Read the model definition and answer for the solid it produces. Units are mm, in the model's axes. Round coordinates to 2 decimals unless told otherwise and drop trailing zeros. Write each loop counter-clockwise with the first axis right and the second up, starting at its lowest first coordinate (ties: lowest second). Pieces come first, ordered by that corner, then holes.
from build123d import *

# Parameters (mm, degrees)
SKETCH1_W           = 76.2
SKETCH1_H           = 288.925
BOSS_EXTRUDE1_DEPTH = 3.175
CUT_EXTRUDE1_REACH  = 300.821
SKETCH2_W           = 65.532
SKETCH2_H           = 96.012


with BuildPart() as part:
    # Sketch1 → Boss-Extrude1 (new body)
    with BuildSketch(Plane(origin=(0, 0, 0), x_dir=(0, 0, -1), z_dir=(1, 0, 0))):
        with Locations((38.1, 144.4625)):
            Rectangle(SKETCH1_W, SKETCH1_H)
    extrude(amount=BOSS_EXTRUDE1_DEPTH)

    # Sketch2 → Cut-Extrude1 (cut, up to next)
    with BuildSketch(Plane.ZY, mode=Mode.PRIVATE) as cut_extrude1_sk1:
        with Locations((-38.1, 234.569)):
            Rectangle(SKETCH2_W, SKETCH2_H)
    cut_extrude1_tool1 = extrude(cut_extrude1_sk1.sketch, amount=-CUT_EXTRUDE1_REACH, mode=Mode.PRIVATE) & part.part
    add(cut_extrude1_tool1.solids().sort_by_distance((0, 234.569, -38.1))[0], mode=Mode.SUBTRACT)


solid = part.part
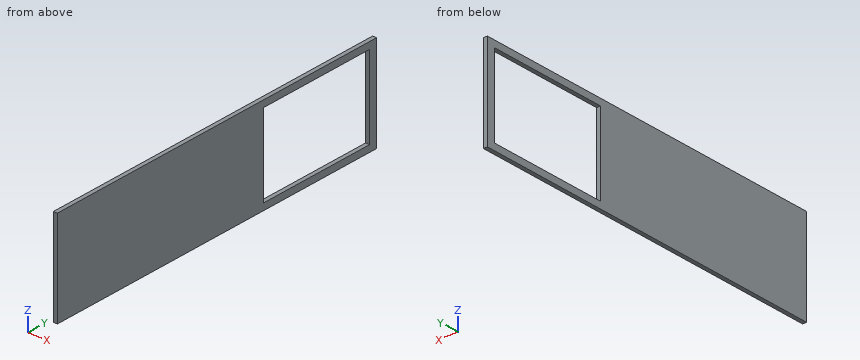
Q1. Section B-B (y = 263.5) is taken. Determine the outline of the cut face in (x, z) (3 decimals).
Verdict:
outline: (0, -76.2) - (3.175, -76.2) - (3.175, -70.866) - (0, -70.866) - close; (0, -5.334) - (3.175, -5.334) - (3.175, 0) - (0, 0) - close
Q2. Section A-A (z = -63) is taken. Determine the outline of the cut face in (x, y) (3 decimals), then the cut area to 4 significant figures.
Verdict:
outline: (0, 0) - (3.175, 0) - (3.175, 186.563) - (0, 186.563) - close; (0, 282.575) - (3.175, 282.575) - (3.175, 288.925) - (0, 288.925) - close
area: 612.5 mm2
Q3. Section C-C (x = 2) is taken. Determine the outline of the cut face in (y, z) (3 decimals).
Verdict:
outline: (0, -76.2) - (288.925, -76.2) - (288.925, 0) - (0, 0) - close; hole (186.563, -70.866) - (282.575, -70.866) - (282.575, -5.334) - (186.563, -5.334) - close
Q4. Straight lines are drawn through the part: probe 1 along Y at (x, z) = (0.6, -68) (3 decimals); probe 2 along Z at (x, y) = (2.25, 264). For each, find the intervals that lie inside material, in ascending order.
Verdict:
probe 1: y = 0 to 186.563, 282.575 to 288.925
probe 2: z = -76.2 to -70.87, -5.33 to 0
